Geometry: final body of the model. Coordinates: model frame, mm. A direction names the side the tool comes from. Give positions to 0.01 mm unless a question says otherwise; leave off trailing zeros. Loops run counter-clockwise (first coordinate to the right, second up) from the corner with the lowest first, then second, coordinate; pieces in that order, holes last.
1. Draft query along Z for faces 1 (the face through (-6, 6, -0.635)), 2 (the face through (-4.08, 1, 5.02)), 3 (the face through (-12.319, 18, 6)). Return one class per face: +Z half, -Z half, draft (parallel to the pull), parting line (faces both ways), or undercut.
2. Access query for faces 4 (the face through (-3, 14.224, 6)), 5 (the face through (-6, 10.668, 4)), 6 (the face through (0, 1, 5)), 7 (the face through (-6, 12.446, 2)), 8 (the face through (-10, 14, 7.049)). Directions: +Z, -Z, +X, -X, +Y, -Y. A direction counts if a zero-diameter tool reaches every point of the face in a straight line with its end or side. Return the directions, or none.
3. Section C-C, the plane x = -18. Output: boundary loops of the cut face in (y, z) (1 decimal).
4. Section D-D, the plane y = 1.5. Output: boundary loops of the cut face in (x, z) (3 decimals).
5. Section A-A, the plane y = 18.5. Output: boundary loops of the cut face in (x, z) (1 decimal).
6. Section B-B, the plane z = 4. Output: boundary loops of the cut face in (x, y) (3 decimals), then the cut area to 3 significant figures.
7. First-contact query: P1, Ø1.5, axis at x = -7, z = 1.5, coming from the +Y side; P2, Ø4.5, axis at x = -7.5, z = 5.5, coming from the -Y side; P3, Ø2, axis at x = -3.175, z = 5.715, coming from the -Y side; P4, Ø2, axis at x = -19, y = 18, coming from the +Z side. Flat tips, straight axial feed; report the tip coordinate or a pass-through.
8. Material intervals for line 1 along Y through (x, z) = (-12.5, 7); line 2 along Y through (x, z) = (-7, 5.25); line 3 along Y through (x, z) = (-0.5, 4), sorted ascending.
from build123d import *

# Parameters (mm, degrees)
F0_W      = 22.225
F0_H      = 8.89
F0_R      = 1.143
F1_DEPTH  = 2.032
F2_W      = 17.78
F2_H      = 1.905
F3_DEPTH  = 22.225
F4_DEPTH  = 10.16
F5_W      = 10.922
F5_H      = 7.6835
F7_DEPTH  = 32.385
F6_W      = 18.288
F6_H      = 3.556
F6_H_2    = 6.604
F8_DEPTH  = 12.7
F9_R      = 1.27
F10_DEPTH = 25.4
F11_W     = 32.385
F11_H     = 9.652
F12_DEPTH = 5.08


with BuildPart() as f1:
    # F0 (on Front) → F1 (new body)
    with BuildSketch(Plane.XZ):
        with Locations((-11.1125, 4.445)):
            Rectangle(F0_W, F0_H)
        with Locations((-15.875, 5.715)):
            Circle(F0_R, mode=Mode.SUBTRACT)
        with Locations((-9.525, 5.715)):
            Circle(F0_R, mode=Mode.SUBTRACT)
        with Locations((-3.175, 5.715)):
            Circle(F0_R, mode=Mode.SUBTRACT)
    extrude(amount=-F1_DEPTH)

    # F2 (on Right) → F3 (join, through all)
    with BuildSketch(Plane.YZ):
        with Locations((8.89, 0.3175)):
            Rectangle(F2_W, F2_H)
    extrude(amount=-F3_DEPTH)

    # F2 (on Right) → F4 (join)
    with BuildSketch(Plane.YZ):
        with Locations((8.89, 0.3175)):
            Rectangle(F2_W, F2_H)
    extrude(amount=F4_DEPTH)

    # F5 (on face) → F7 (join, through all)
    with BuildSketch(Plane(origin=(-22.225, 0, 0), x_dir=(0, -1, 0), z_dir=(-1, 0, 0))):
        with Locations((-16.129, 3.20675)):
            Rectangle(F5_W, F5_H)
    extrude(amount=-F7_DEPTH)

    # F6 (on face) → F8 (cut, symmetric)
    with BuildSketch(Plane.XY.offset(1.27)):
        with Locations((-3.175, 16.002)):
            Rectangle(F6_W, F6_H)
        with Locations((-3.175, 21.082)):
            Rectangle(F6_W, F6_H_2)
    extrude(amount=F8_DEPTH, both=True, mode=Mode.SUBTRACT)

    # F9 (on face) → F10 (cut)
    with BuildSketch(Plane.XY.offset(7.0485)):
        with Locations((-13.462, 14.605)):
            Circle(F9_R)
        with Locations((7.112, 14.605)):
            Circle(F9_R)
    extrude(amount=-F10_DEPTH, mode=Mode.SUBTRACT)

    # F11 (on face) → F12 (cut)
    with BuildSketch(Plane(origin=(0, 0, -0.635), x_dir=(1, 0, 0), z_dir=(0, 0, -1))):
        with Locations((-6.0325, -17.272)):
            Rectangle(F11_W, F11_H)
    extrude(amount=-F12_DEPTH, mode=Mode.SUBTRACT)


solid = f1.part
Answers below:
1. face 1: -Z half
1. face 2: undercut
1. face 3: draft
2. face 4: +Z, -Z, +Y
2. face 5: +Z, +X, -X
2. face 6: +Z, +X, -Y
2. face 7: -Z, +X, -X, +Y
2. face 8: +Z, +X, -X, +Y
3. outline: (0, -0.6) - (12.4, -0.6) - (12.4, 4.4) - (21.6, 4.4) - (21.6, 7) - (10.7, 7) - (10.7, 1.3) - (2, 1.3) - (2, 8.9) - (0, 8.9) - close
4. outline: (-22.225, -0.635) - (10.16, -0.635) - (10.16, 1.27) - (0, 1.27) - (0, 8.89) - (-22.225, 8.89) - close; hole circle Ø2.286 at (-15.875, 5.715); hole circle Ø2.286 at (-9.525, 5.715); hole circle Ø2.286 at (-3.175, 5.715)
5. outline: (-22.2, 4.4) - (-12.3, 4.4) - (-12.3, 7) - (-22.2, 7) - close; (6, 4.4) - (10.2, 4.4) - (10.2, 7) - (6, 7) - close
6. outline: (-22.225, 0) - (0, 0) - (0, 2.032) - (-22.225, 2.032) - close; (-22.225, 10.668) - (10.16, 10.668) - (10.16, 12.446) - (-22.225, 12.446) - close
6. area: 103 mm2
7. P1: stops at y = 12.45
7. P2: stops at y = 0
7. P3: stops at y = 10.67
7. P4: stops at z = 7.05
8. line 1: y = 0 to 2.03, 10.67 to 13.78, 15.43 to 21.59
8. line 2: y = 0 to 2.03, 10.67 to 14.22
8. line 3: y = 0 to 2.03, 10.67 to 12.45
